from build123d import *

# Parameters (mm, degrees)
F0_W     = 75
F0_H     = 120
F0_R     = 2
F0_W_2   = 11
F0_H_2   = 25
F1_DEPTH = 5.5
F2_R     = 4
F3_R     = 2


with BuildPart() as f1:
    # F0 (on Front) → F1 (new body)
    with BuildSketch(Plane.XZ):
        Rectangle(F0_W, F0_H)
        with Locations((0, -30)):
            Circle(F0_R, mode=Mode.SUBTRACT)
        Rectangle(F0_W_2, F0_H_2, mode=Mode.SUBTRACT)
        with Locations((0, 30)):
            Circle(F0_R, mode=Mode.SUBTRACT)
    extrude(amount=F1_DEPTH)

    # F2
    f2_edges = [f1.edges().sort_by_distance(p)[0] for p in [
        (-37.5, -5.5, 0),
        (0, -5.5, 60),
        (37.5, -5.5, 0),
        (0, -5.5, -60),
    ]]
    fillet(f2_edges, radius=F2_R)

    # F3
    f3_edges = [f1.edges().sort_by_distance(p)[0] for p in [
        (-2, -5.5, 30),
        (-2, -5.5, -30),
    ]]
    fillet(f3_edges, radius=F3_R)


solid = f1.part
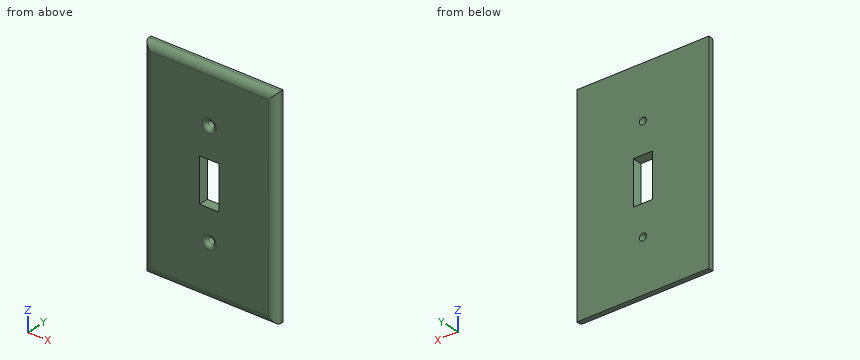
Work out the finished part from the listing and answer in its coordinate system (mm). Give positions to 0.01 mm unless a question says otherwise; leave off trailing zeros. Write each loop counter-clockwise with the first axis right and the second up, starting at its lowest first coordinate (ties: lowest second). Pieces come first, ordered by that corner, then holes. Notation, with made-up numbers: (66.25, 5.25) - (70.25, 5.25) arc R23 cw to (70.25, 41.25) - close; hole circle Ø11 at (45.5, 88). An arc over 180 degrees is marked (long way). One line per item, written item: value. Start each with the question number.
1. Find section D-D (z = -17). Write down the section's boundary in (x, y).
2. Find section C-C (y = -2.4). Write down the section's boundary in (x, z).
3. Find section B-B (z = -30). Write down the section's boundary in (x, y), then the cut area to 3 significant figures.
4. Given pin 1 (3 mm diameter, centred on x = 0, z = -30, fed in from -Y); pin 2 (1 mm diameter, centred on x = -27.5, y = -4.5, fed in from +Z); pin 3 (1 mm diameter, centred on x = 13, y = -4, fed in from +Z); pin 4 (1.5 mm diameter, centred on y = -2.5, z = 23.5, fed in from +X), each flat-ended and moving along its own axis, determine where each tip first touches the part or whether it passes through.
5. Find section A-A (x = 0). Write down the section's boundary in (y, z).
6. Consider probe 1 along Z at (x, y) = (0, -1.35); probe 2 along Z at (x, y) = (0, -2.35); probe 3 along X at (y, z) = (-1.95, -8). Determine where each line is inside the solid, lowest interval first.
Geometry results:
1. outline: (-37.5, -1.5) arc R4 ccw to (-33.5, -5.5) - (33.5, -5.5) arc R4 ccw to (37.5, -1.5) - (37.5, 0) - (-37.5, 0) - close
2. outline: (-37.4, -59.9) - (37.4, -59.9) - (37.4, 59.9) - (-37.4, 59.9) - close; hole (-5.5, -12.5) - (5.5, -12.5) - (5.5, 12.5) - (-5.5, 12.5) - close; hole circle Ø4 at (0, -30); hole circle Ø4 at (0, 30)
3. outline: (-37.5, -1.5) arc R4 ccw to (-33.5, -5.5) - (-4, -5.5) arc R2 ccw to (-2, -3.5) - (-2, 0) - (-37.5, 0) - close; (2, -3.5) arc R2 ccw to (4, -5.5) - (33.5, -5.5) arc R4 ccw to (37.5, -1.5) - (37.5, 0) - (2, 0) - close
3. area: 382 mm2
4. pin 1: through
4. pin 2: z = 59.12
4. pin 3: z = 59.46
4. pin 4: x = 37.49
5. outline: (-5.5, -56) arc R4 ccw to (-1.5, -60) - (0, -60) - (0, -32) - (-3.5, -32) arc R2 ccw to (-5.5, -34) - close; (-5.5, -26) arc R2 ccw to (-3.5, -28) - (0, -28) - (0, -12.5) - (-5.5, -12.5) - close; (-5.5, 12.5) - (0, 12.5) - (0, 28) - (-3.5, 28) arc R2 ccw to (-5.5, 26) - close; (-5.5, 34) arc R2 ccw to (-3.5, 32) - (0, 32) - (0, 60) - (-1.5, 60) arc R4 ccw to (-5.5, 56) - close
6. probe 1: -60 to -32, -28 to -12.5, 12.5 to 28, 32 to 60
6. probe 2: -59.91 to -32, -28 to -12.5, 12.5 to 28, 32 to 59.91
6. probe 3: -37.47 to -5.5, 5.5 to 37.47
